Geometry: final body of the model. Coordinates: model frame, mm. A direction names the side the tool comes from. Coordinates: 2 decimals unless noted, no trailing zeros. Loops run counter-clockwise (first coordinate to the right, second up) from the corner with the lowest first, then second, coordinate; pieces in that order, holes last. Notation, with made-up numbers: (32, 46) - (89, 46) arc R19 cw to (89, 70) - close; hole circle Ø11 at (82.25, 61). An arc over 180 degrees is marked (long way). Put each result on its own line as item: value. Start each with the question number.
1) Section A-A on x = 0. Output: boundary loops of the cut face in (y, z), and give its area (3 significant figures).
2) Reachability of faces 1 (the flat face through (23, 5, 23)), 2 (the cylindrical face through (7.7, 0.1, 10.1)), 3 (the cylindrical face through (27.041, -7.535, 6.005)) from +Z, -Z, +X, -X, +Y, -Y: full face, straight path, thin tool, end or side. Return the list, or none.
3) Contact query for flat-ended pins moving along their axis: pin 1 Ø4 at (y, z) = (-5.5, -46) entering from +X; pin 2 Ø4 at (x, y) = (-41, -4) entering from -Z; pin 3 Ø1 at (y, z) = (8, 26.5) entering from +X; pin 4 Ø20.5 at (x, z) = (0, 0) entering from +Y. Output: stop coordinate, or through.
4) Section B-B on z = 0. Output: boundary loops of the cut face in (x, y).
5) Section C-C on y = -6.75. Output: boundary loops of the cut face in (x, z).
6) Draft query along X for faces 4 (the flat face through (23, -5, -23)), 5 (the flat face through (6, 10, 12)). Return one class per face: +X half, -X half, draft (parallel to the pull), parting line (faces both ways), or undercut.
7) Material intervals for line 1 along X through (y, z) = (8.5, 0); line 2 along X through (y, z) = (6.6, 0); line 3 along Y through (x, z) = (41, -9), sorted ascending. Write a range as from..to.
```python
from build123d import *


with BuildPart() as part:
    # Croquis1 → Revolución1 (revolve)
    with BuildSketch(Plane.XY, mode=Mode.PRIVATE) as revoluci_n1_sk:
        with BuildLine():
            Line((12.7, -10), (12.7, 10))
            Line((12.7, 10), (27.7, 10))
            Line((27.7, 10), (27.7, 5))
            Line((27.7, 5), (52.7, 5))
            Line((52.7, 5), (52.7, 10))
            Line((52.7, 10), (60, 10))
            ThreePointArc((60, 10), (70, 0), (60, -10))
            Line((60, -10), (52.7, -10))
            Line((52.7, -10), (52.7, -5))
            Line((52.7, -5), (27.7, -5))
            Line((27.7, -5), (27.7, -10))
            Line((27.7, -10), (12.7, -10))
        make_face()
    revolve(revoluci_n1_sk.sketch.rotate(Axis((0, 0, 0), (0, 1, 0)), 90), axis=Axis((0, 0, 0), (0, 1, 0)))


solid = part.part
```
Answer block:
1. outline: (-10, -60) arc R10 ccw to (10, -60) - (10, -52.7) - (5, -52.7) - (5, -27.7) - (10, -27.7) - (10, -12.7) - (-10, -12.7) - (-10, -27.7) - (-5, -27.7) - (-5, -52.7) - (-10, -52.7) - close; (-10, 12.7) - (10, 12.7) - (10, 27.7) - (5, 27.7) - (5, 52.7) - (10, 52.7) - (10, 60) arc R10 ccw to (-10, 60) - (-10, 52.7) - (-5, 52.7) - (-5, 27.7) - (-10, 27.7) - close
1. area: 1,710 mm²
2. face 1: +Y
2. face 2: +Y, -Y
2. face 3: -Y
3. pin 1: stops at x = 52.85
3. pin 2: stops at z = -57.39
3. pin 3: stops at x = 61.15
3. pin 4: passes through
4. outline: (-60, -10) - (-52.7, -10) - (-52.7, -5) - (-27.7, -5) - (-27.7, -10) - (-12.7, -10) - (-12.7, 10) - (-27.7, 10) - (-27.7, 5) - (-52.7, 5) - (-52.7, 10) - (-60, 10) arc R10 ccw to start; (12.7, -10) - (27.7, -10) - (27.7, -5) - (52.7, -5) - (52.7, -10) - (60, -10) arc R10 ccw to (60, 10) - (52.7, 10) - (52.7, 5) - (27.7, 5) - (27.7, 10) - (12.7, 10) - close
5. outline: circle Ø134.76 at (0, 0); circle Ø55.4 at (0, 0); hole circle Ø105.4 at (0, 0); hole circle Ø25.4 at (0, 0)
6. face 4: undercut
6. face 5: draft
7. line 1: x = -65.27..-52.7, -27.7..-12.7, 12.7..27.7, 52.7..65.27
7. line 2: x = -67.51..-52.7, -27.7..-12.7, 12.7..27.7, 52.7..67.51
7. line 3: y = -5..5
